```python
from build123d import *

# Parameters (mm, degrees)
SKETCH_1_W          = 180
SKETCH_1_H          = 63
EXTRUDE_1_DEPTH     = 5
SKETCH_2_R          = 2.1
CUT_EXTRUDE_1_DEPTH = 5
CUT_EXTRUDE_2_DEPTH = 200
SKETCH_5_W          = 180
SKETCH_5_H          = 30.5
EXTRUDE_2_DEPTH     = 5
SKETCH_7_R          = 2.1
CUT_EXTRUDE_3_DEPTH = 5
FILLET_3_R          = 9
FILLET_4_R          = 7
SKETCH_8_W          = 120
SKETCH_8_H          = 50
CUT_EXTRUDE_4_DEPTH = 5
FILLET_5_R          = 5


with BuildPart() as part:
    # 草图1 → 凸台-拉伸1 (new body)
    with BuildSketch(Plane(origin=(0, 0, 0), x_dir=(1, 0, 0), z_dir=(0, 1, 0))):
        Rectangle(SKETCH_1_W, SKETCH_1_H)
    extrude(amount=EXTRUDE_1_DEPTH)

    # 草图2 → 切除-拉伸1 (cut)
    with BuildSketch(Plane(origin=(0, 5, 0), x_dir=(1, 0, 0), z_dir=(0, 1, 0))):
        with Locations(Location((80, 23.27, 0), (0, 0, 270))):
            Circle(SKETCH_2_R)
        with Locations(Location((80, 8.34, 0), (0, 0, 270))):
            Circle(SKETCH_2_R)
        with Locations(Location((80, -6.59, 0), (0, 0, 270))):
            Circle(SKETCH_2_R)
        with Locations(Location((-80, 23.27, 0), (0, 0, 90))):
            Circle(SKETCH_2_R)
        with Locations(Location((-80, 8.34, 0), (0, 0, 90))):
            Circle(SKETCH_2_R)
        with Locations(Location((-80, -6.59, 0), (0, 0, 90))):
            Circle(SKETCH_2_R)
    extrude(amount=-CUT_EXTRUDE_1_DEPTH, mode=Mode.SUBTRACT)

    # 草图3 → 切除-拉伸2 (cut)
    with BuildSketch(Plane.ZY.offset(90)):
        Polygon((26.5, 5), (29.386751346, 0), (31.5, 0), (31.5, 5), align=None)
    extrude(amount=-CUT_EXTRUDE_2_DEPTH, mode=Mode.SUBTRACT)

    # 草图5 → 凸台-拉伸2 (add)
    with BuildSketch(Plane(origin=(0, 12.7248366, 22.040063509), x_dir=(1, 0, 0), z_dir=(0, 0.49999999999999806, 0.8660254037844399))):
        with Locations((0, -24.169872981)):
            Rectangle(SKETCH_5_W, SKETCH_5_H)
    extrude(amount=EXTRUDE_2_DEPTH)

    # 草图7 → 切除-拉伸3 (cut)
    with BuildSketch(Plane(origin=(0, 15.2248366, 26.370190528), x_dir=(1, 0, 0), z_dir=(0, 0.4999999999999981, 0.8660254037844397))):
        with Locations(Location((37.5, -24.419872981, 0), (0, 0, 270))):
            Circle(SKETCH_7_R)
        with Locations(Location((-37.5, -24.419872981, 0), (0, 0, 90))):
            Circle(SKETCH_7_R)
    extrude(amount=-CUT_EXTRUDE_3_DEPTH, mode=Mode.SUBTRACT)

    # 圆角3
    # the kernel refuses this fillet: 9 mm, written as the material it takes off along each edge
    with BuildSketch(Plane(origin=(110.155644371, 7.5, 30.830127019), x_dir=(0, -0.8660254037844398, 0.499999999999998), z_dir=(-1, 0, 0))) as fillet_3_piece_1:
        with BuildLine():
            CenterArc((8.062257748, -9), FILLET_3_R, 90, 63.612200039)
            Line((0, -5), (-0.161245155, -4.92))
            ThreePointArc((-0.161245155, -4.92), (-0.18, -2.5), (-0.18, 0))
            Line((-0.18, 0), (0, 0.18))
            Line((0, 0.18), (8.062257748, 0.18))
            Line((8.062257748, 0.18), (8.062257748, 0))
        make_face()
    extrude(amount=220.311288741, mode=Mode.SUBTRACT)

    # 圆角4
    fillet_4_edges = [part.edges().sort_by_distance(p)[0] for p in [
        (0, 0, 29.386751346),
    ]]
    fillet(fillet_4_edges, radius=FILLET_4_R)

    # 草图8 → 切除-拉伸4 (cut)
    with BuildSketch(Plane(origin=(0, 5, 0), x_dir=(1, 0, 0), z_dir=(0, 1, 0))):
        with Locations((0, 8.5)):
            Rectangle(SKETCH_8_W, SKETCH_8_H)
    extrude(amount=-CUT_EXTRUDE_4_DEPTH, mode=Mode.SUBTRACT)

    # 圆角5
    fillet_5_edges = [part.edges().sort_by_distance(p)[0] for p in [
        (60, 2.5, -31.5),
        (-60, 2.5, -31.5),
        (-60, 2.5, 16.5),
        (60, 2.5, 16.5),
        (-90, 2.5, -31.5),
        (90, 2.5, -31.5),
    ]]
    fillet(fillet_5_edges, radius=FILLET_5_R)


solid = part.part
```
Could you check a few things on this model? Use its own coordinates, in mm. A direction names the side the tool comes from. Give positions to 0.01 mm unless a question says otherwise; leave off trailing zeros. Loops run counter-clockwise (first coordinate to the right, second up) from the corner with the lowest first, then second, coordinate; pieces in that order, holes last. Notation, with made-up numbers: (33.5, 47) -> (52.5, 47) arc R14 cw to (52.5, 68) -> close; hole circle Ø4 at (-7.5, 46). An arc over 180 degrees is marked (long way). Put each result on its own line as item: value.
(1) Imagine slicing it at C-C on z = -14.5. Write out the boundary of the cut face in (x, y).
Computed:
outline: (-90, 0) -> (-60, 0) -> (-60, 5) -> (-90, 5) -> close; (60, 0) -> (90, 0) -> (90, 5) -> (60, 5) -> close
(2) Imagine slicing it at A-A on x = 80. Write out the boundary of the cut face in (y, z), plus the area to 3 significant figures.
Computed:
outline: (-21.41, 41.75) -> (-3.5, 31.41) arc R7 cw to (0, 25.35) -> (0, 8.69) -> (5, 8.69) -> (5, 26.5) arc R9 ccw to (0.52, 34.86) -> (-18.91, 46.08) -> close; (0, -31.5) -> (5, -31.5) -> (5, -25.37) -> (0, -25.37) -> close; (0, -21.17) -> (5, -21.17) -> (5, -10.44) -> (0, -10.44) -> close; (0, -6.24) -> (5, -6.24) -> (5, 4.49) -> (0, 4.49) -> close
area: 378 mm^2
(3) For faces 1 (the face through (61.43, 2.46, -30)), 2 (the face through (90, 2, 12)), which set-ups out of +Z, -Z, +X, -X, +Y, -Y let a thin tool reach every point of the face, with its end or its side?
Computed:
face 1: -Z, +Y, -Y
face 2: +Z, -Z, +X, +Y, -Y
(4) Please list where these lines run through material, in increasing order: probe 1 along X at (y, z) = (2.4, -8.34); probe 2 along Z at (x, y) = (-80, 3.15); probe 3 along Z at (x, y) = (-80, 3.9). Write a range as [from, to].
Computed:
probe 1: [-90, -82.1], [-77.9, -60], [60, 77.9], [82.1, 90]
probe 2: [-31.5, -25.37], [-21.17, -10.44], [-6.24, 4.49], [8.69, 32.56]
probe 3: [-31.5, -25.37], [-21.17, -10.44], [-6.24, 4.49], [8.69, 31.41]
(5) I'm going to push flat-ended pins straight in: pin 1 Ø12 at (y, z) = (-8.5, -4) entering from -X; pin 2 Ø6 at (x, z) = (-50.5, 17) entering from +Y; pin 3 Ø2.5 at (x, y) = (12, 2.5) entering from -Z; pin 4 Ø8 at (x, y) = (53, 1) entering from +Z. Where does each tip first touch, or does it pass through?
Computed:
pin 1: through
pin 2: y = 5
pin 3: z = 16.5
pin 4: z = 36.89
(6) Thinking about a two-plate mould opening in X: for faces 3 (the face through (88.57, 2.54, -30)), 4 (the face through (-58.57, 2.46, 15)), 5 (the face through (-88.57, 2.54, -30)), which applies, pulls with the +X half, pulls with the -X half, needs draft (parallel to the pull), parting line crosses it, or undercut?
Computed:
face 3: pulls with the +X half
face 4: undercut
face 5: pulls with the -X half
(7) Imagine slicing it at D-D on x = -26. Write out the boundary of the cut face in (y, z), plus the area to 3 significant figures.
Computed:
outline: (-21.41, 41.75) -> (-3.5, 31.41) arc R7 cw to (0, 25.35) -> (0, 16.5) -> (5, 16.5) -> (5, 26.5) arc R9 ccw to (0.52, 34.86) -> (-18.91, 46.08) -> close
area: 201 mm^2
(8) Imagine slicing it at B-B on z = 6.59. Write out the boundary of the cut face in (x, y).
Computed:
outline: (-90, 0) -> (-82.1, 0) -> (-82.1, 5) -> (-90, 5) -> close; (-77.9, 0) -> (-60, 0) -> (-60, 5) -> (-77.9, 5) -> close; (60, 0) -> (77.9, 0) -> (77.9, 5) -> (60, 5) -> close; (82.1, 0) -> (90, 0) -> (90, 5) -> (82.1, 5) -> close
